```python
from build123d import *

# Parameters (mm, degrees)
BOSS_EXTRUDE1_DEPTH = 8
SKETCH2_R           = 2.4
BOSS_EXTRUDE2_DEPTH = 1.6
SHELL1_T            = -1.6


with BuildPart() as part:
    # Sketch1 → Boss-Extrude1 (new body)
    with BuildSketch(Plane(origin=(0, 0, 0), x_dir=(0, 0, -1), z_dir=(1, 0, 0))):
        Polygon((0, 0), (16, 0), (8, 9.6), (0, 9.6), align=None)
    extrude(amount=BOSS_EXTRUDE1_DEPTH)

    # Sketch2 → Boss-Extrude2 (add)
    with BuildSketch(Plane(origin=(0, 9.6, 0), x_dir=(1, 0, 0), z_dir=(0, 1, 0))):
        with Locations(Location((4, 4, 0), (0, 0, 270))):
            Circle(SKETCH2_R)
    extrude(amount=BOSS_EXTRUDE2_DEPTH)

    # Shell1
    shell1_openings = [part.faces().sort_by_distance(p)[0] for p in [
        (4, 0, -8),
    ]]
    offset(amount=SHELL1_T, openings=shell1_openings, kind=Kind.INTERSECTION)


solid = part.part
```
Read the model definition and answer for the solid it produces. Units are mm, in the model's axes. A direction names the side the tool comes from. Give positions to 0.01 mm unless a question says otherwise; leave off trailing zeros. Order: outer loops, then holes, each group sorted by start corner. A loop starts at its lowest first (then second) coordinate and runs counter-clockwise, first axis right, second up.
(1) Find section B-B (z = -4). Give the vertices of the cut face in (x, y).
(2) Straight lines are drawn through the part: L1, parallel to X at y = 2, z = -9.5; L2, parallel to X at y = 8.4, z = -4; L3, parallel to Y at x = 1, z = -3.25. For each, find the intervals that lie inside material, in ascending order.
(3) For a pull along X with two mould halves and no side action, classify faces 4 (the flat face through (6, 9.6, -2)), 5 (the flat face through (8, 5, -6)), 6 (the flat face through (1.6, 3, -6)) as released by +X, released by -X, zero draft, split by the parting line, or undercut.
(4) Find section A-A (y = 6.25). Give the vertices of the cut face in (x, z), plus the area to 3 significant figures.
(5) For faces 1 (the cylindrical face through (6.024, 10.389, -2.71)), 2 (the flat face through (4, 4, -1.6)), 3 (the flat face through (7, 0, -8)), determine the directions among +Z, -Z, +X, -X, +Y, -Y from which every point of the face is accessible in a straight line to the end or side of a thin tool.
(6) Given pin 1 (2 mm diameter, centred on x = 6.5, z = -10, fed in from +Y); pin 2 (1.3 mm diameter, centred on x = 3.5, z = -4.5, fed in from -Y); pin 3 (2.5 mm diameter, centred on x = 4.5, y = 6, fed in from -Z), each flat-ended and moving along its own axis, determine where each tip first touches the part or whether it passes through.
(7) Find section C-C (x = 4). Give the vertices of the cut face in (y, z), plus the area to 3 significant figures.
(8) Find section D-D (y = 10.5). Give the vertices of the cut face in (x, z).
Result sheet:
1. outline: (0, 0) - (1.6, 0) - (1.6, 8) - (3.2, 8) - (3.2, 9.6) - (4.8, 9.6) - (4.8, 8) - (6.4, 8) - (6.4, 0) - (8, 0) - (8, 9.6) - (6.4, 9.6) - (6.4, 11.2) - (1.6, 11.2) - (1.6, 9.6) - (0, 9.6) - close
2. L1: x = 0 to 1.6, 6.4 to 8
2. L2: x = 0 to 3.2, 4.8 to 8
2. L3: y = 0 to 9.6
3. face 4: zero draft
3. face 5: released by +X
3. face 6: undercut
4. outline: (0, -10.79) - (8, -10.79) - (8, 0) - (0, 0) - close; hole (1.6, -8.71) - (6.4, -8.71) - (6.4, -1.6) - (1.6, -1.6) - close
4. area: 52.2 mm2
5. face 1: +Y
5. face 2: -Y
5. face 3: +Z, -Z, +X, -X, -Y
6. pin 1: stops at y = 8.4
6. pin 2: stops at y = 8
6. pin 3: stops at z = -12.04
7. outline: (0, -16) - (9.6, -8) - (9.6, -6.4) - (11.2, -6.4) - (11.2, -1.6) - (9.6, -1.6) - (9.6, 0) - (0, 0) - (0, -1.6) - (8, -1.6) - (8, -3.2) - (9.6, -3.2) - (9.6, -4.8) - (8, -4.8) - (8, -7.25) - (0, -13.92) - close
7. area: 48.4 mm2
8. outline: circle Ø4.8 at (4, -4)
